Check sheet for the drawn part. Datum: minimum x, y, z corner. Units: mm. A direction names the side the tool comes from. Round coordinates to 2 decimals unless told otherwise and drop trailing zeros. Order: outer loops, then holes, each group sorted by start corner. A loop starts at its lowest first (then second) coordinate and runs counter-clockwise, first axis right, second up. Notation, with made-up numbers: (79, 50.25) -> (115, 50.25) arc R32 cw to (115, 88.25) -> close; hole circle Ø9 at (36.5, 34.5). An arc over 180 degrees is marked (long way). Answer in a Markdown table with one row per item.
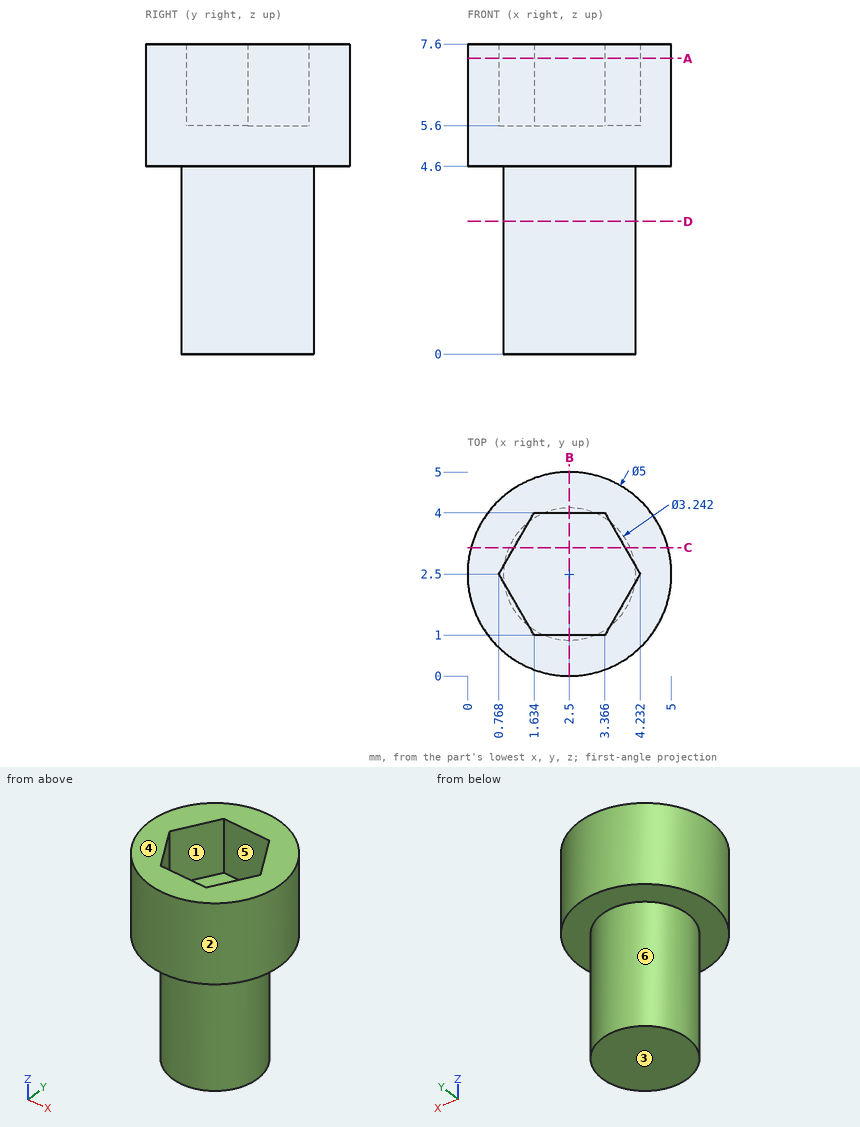
(1) Tool access check on the marked faces 4, 5 and 6. Record the directions out of +Z, -Z, +X, -X, +Y, -Y that give a thin tool (end or side, any length) a straight path to the whole face; none if there is none.
Solutions:
| item | result |
|---|---|
| face 4 | +Z, +X, -X, +Y, -Y |
| face 5 | +Z |
| face 6 | -Z |
(2) Scan lines: probe 1 along Z at (x, y) = (3, 3.95); probe 2 along Z at (x, y) = (0.75, 1.05); probe 3 along X at (y, z) = (2.55, 0.5). Record each from-to range of solid material in increasing order. Write a range as from..to.
Solutions:
| item | result |
|---|---|
| probe 1 | 0..5.6 |
| probe 2 | 4.6..7.6 |
| probe 3 | 0.88..4.12 |
(3) Section check C-C on y = 3.15. Record the boundary of the cut face in (x, z) (3 decimals).
Solutions:
| item | result |
|---|---|
| outline | (0.086, 4.6) -> (1.015, 4.6) -> (1.015, 0) -> (3.985, 0) -> (3.985, 4.6) -> (4.914, 4.6) -> (4.914, 7.6) -> (3.857, 7.6) -> (3.857, 5.6) -> (1.143, 5.6) -> (1.143, 7.6) -> (0.086, 7.6) -> close |
(4) Draft check along X on the marked faces 1, 2 and 3. Enter one of: pulls with the +X half, pulls with the -X half, needs draft (parallel to the pull), parting line crosses it, or undercut.
Solutions:
| item | result |
|---|---|
| face 1 | undercut |
| face 2 | parting line crosses it |
| face 3 | needs draft |
(5) Section check D-D on z = 3.25. Record the boundary of the cut face in (x, y).
Solutions:
| item | result |
|---|---|
| outline | circle Ø3.24 at (2.5, 2.5) |
(6) Section check B-B on x = 2.5. Record the boundary of the cut face in (y, z).
Solutions:
| item | result |
|---|---|
| outline | (0, 4.6) -> (0.88, 4.6) -> (0.88, 0) -> (4.12, 0) -> (4.12, 4.6) -> (5, 4.6) -> (5, 7.6) -> (4, 7.6) -> (4, 5.6) -> (1, 5.6) -> (1, 7.6) -> (0, 7.6) -> close |
(7) Depth check by flat-ended pin: pin 1 Ø0.5 at (x, z) = (3, 7) entering from -Y; pin 2 Ø1.5 at (x, y) = (1, 3.5) entering from -Z; pin 3 Ø1 at (y, z) = (3.5, 5) entering from -X; pin 4 Ø1 at (x, z) = (3.5, 3) entering from -Y. Enter the tip coordinate at first touch or a pass-through.
Solutions:
| item | result |
|---|---|
| pin 1 | y = 0.01 |
| pin 2 | z = 0 |
| pin 3 | x = 0.05 |
| pin 4 | y = 0.96 |
(8) Section check A-A on z = 7.25. Record the boundary of the cut face in (x, y).
Solutions:
| item | result |
|---|---|
| outline | circle Ø5 at (2.5, 2.5); hole (0.77, 2.5) -> (1.63, 1) -> (3.37, 1) -> (4.23, 2.5) -> (3.37, 4) -> (1.63, 4) -> close |
